from build123d import *

# Parameters (mm, degrees)
BOSS_EXTRUDE1_DEPTH = 5.588
FILLET1_R           = 25.4
BOSS_EXTRUDE2_DEPTH = 5.588
FILLET2_R           = 6.35
FILLET3_R           = 33.528


with BuildPart() as part:
    # Sketch1 → Boss-Extrude1 (new body)
    with BuildSketch(Plane(origin=(0, 0, 0), x_dir=(1, 0, 0), z_dir=(0, 1, 0))):
        with BuildLine():
            Line((0, 0), (214.63, 0))
            Line((214.63, 0), (214.63, 73.66))
            ThreePointArc((214.63, 73.66), (184.284533276, 157.475694397), (107.315, 202.438))
            ThreePointArc((107.315, 202.438), (30.345466724, 157.475694397), (0, 73.66))
            Line((0, 73.66), (0, 0))
        make_face()
    extrude(amount=BOSS_EXTRUDE1_DEPTH)

    # Fillet1
    fillet1_edges = [part.edges().sort_by_distance(p)[0] for p in [
        (107.315, 2.794, -202.438),
    ]]
    fillet(fillet1_edges, radius=FILLET1_R)

    # Sketch2 → Boss-Extrude2 (add)
    with BuildSketch(Plane(origin=(0, 5.588, 0), x_dir=(1, 0, 0), z_dir=(0, 1, 0))):
        with BuildLine():
            Line((138.43, 0), (76.2, 0))
            ThreePointArc((76.2, 0), (107.315, -20.32), (138.43, 0))
        make_face()
    extrude(amount=-BOSS_EXTRUDE2_DEPTH)

    # Fillet2
    fillet2_edges = [part.edges().sort_by_distance(p)[0] for p in [
        (76.2, 2.794, 0),
        (138.43, 2.794, 0),
    ]]
    fillet(fillet2_edges, radius=FILLET2_R)

    # Fillet3
    fillet3_edges = [part.edges().sort_by_distance(p)[0] for p in [
        (214.63, 2.794, 0),
        (0, 2.794, 0),
    ]]
    fillet(fillet3_edges, radius=FILLET3_R)


solid = part.part
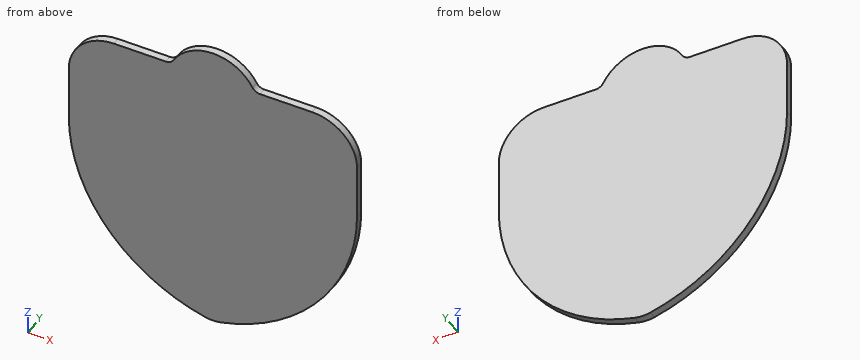
Geometry: final body of the model. Coordinates: model frame, mm. Round coordinates to 2 decimals unless told otherwise and drop trailing zeros. Order: outer loops, then holes, each group sorted by start corner. A loop starts at its lowest first (then second) coordinate and runs counter-clockwise, first axis right, second up. Notation, with made-up numbers: (28.25, -40) - (50.25, -40) arc R29 cw to (50.25, -5) - close; hole circle Ø10 at (-6, 49.25). An arc over 180 degrees is marked (long way). Write each question's results on one line, items separated by ' | '.
Item 1: Section A-A, the plane x = 48. Return the cut outline in (y, z).
Completed:
outline: (0, -174.98) - (5.59, -174.98) - (5.59, 0) - (0, 0) - close
Item 2: Section B-B, the plane z = -149.5. Return the cut outline in (x, y), and give its area (3 significant figures).
Completed:
outline: (24.2, 0) - (190.43, 0) - (190.43, 5.59) - (24.2, 5.59) - close | area: 929 mm^2
Item 3: Material intervals for line 1 along X through (y, z) = (3.05, -164.5); line 2 along X through (y, z) = (2.6, -96.5); line 3 along Z through (x, y) = (155, 5.35), sorted ascending. Write a range as [from, to].
Completed:
line 1: [36.64, 177.99] | line 2: [2.01, 212.62] | line 3: [-183.47, 0]
Item 4: First-contact query: pin 1 Ø1 at (y, z) = (4, -177.5) entering from -X; pin 2 Ø3 at (y, z) = (1, -116) entering from +X; pin 3 Ø1 at (x, y) = (88, 4.5) entering from -Z. Flat tips, straight axial feed; report the tip coordinate or a pass-through.
Completed:
pin 1: x = 50.54 | pin 2: x = 208.1 | pin 3: z = -197.52
